Geometry: see drawing. Coordinates: mm, zero at the bounding-box minimum. A direction names the side the tool comes from. Give positions to 0.01 mm unless a question says otherwise; leave off trailing zeros. Write each loop counter-clockwise with the first axis right and the second up, starting at its lowest first coordinate (ties: lowest second). Pieces come first, ordered by that corner, then holes. Notation, with made-up numbers: (20.25, 78.25) -> (52.25, 78.25) arc R20 ccw to (52.25, 106.25) -> close; hole circle Ø10 at (-18.75, 57.5). An arc over 180 degrees is marked (long way). Answer as a JSON object with one key per item and string values. Group by question number.
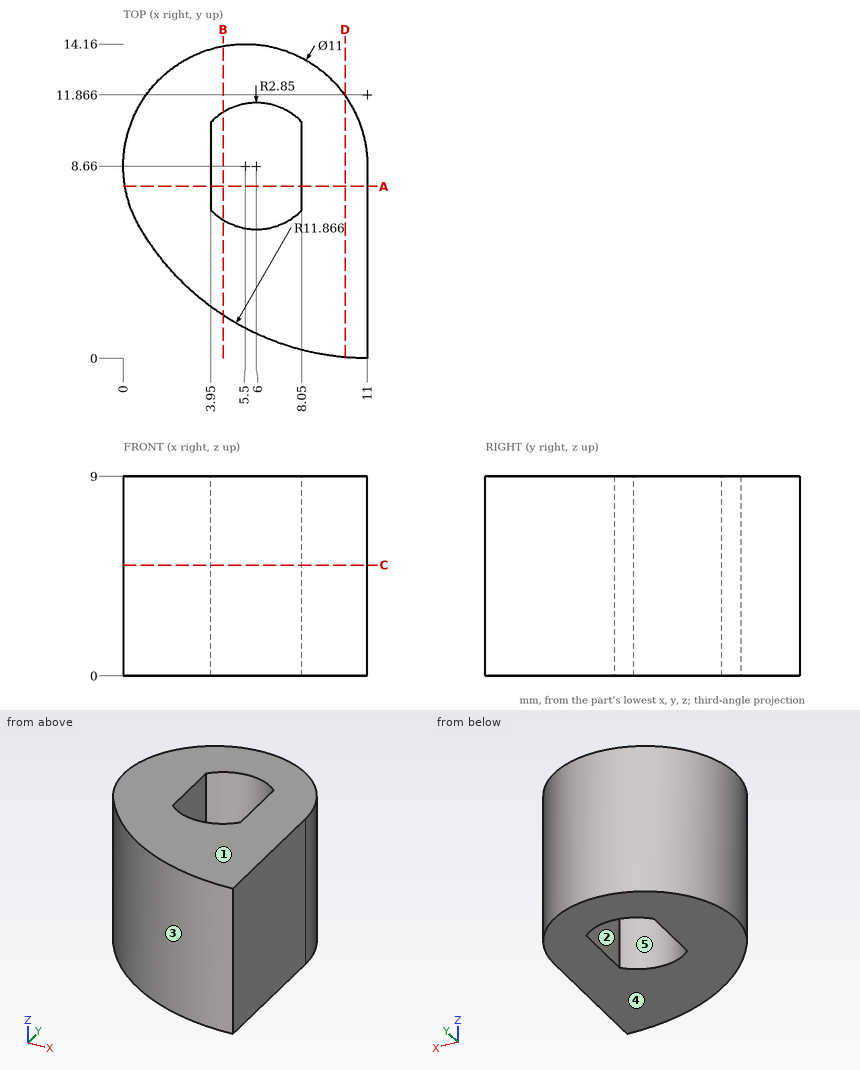
1. Section B-B (x = 4.5). Return the cut outline in (y, z).
2. Section A-A (y = 7.75). Return the cut outline in (x, z).
3. Section D-D (x = 10). Return the cut outline in (y, z), plus the area to 3 significant figures.
4. Reachability of the marked faces 4 and 5 from +Z, -Z, +X, -X, +Y, -Y: full face, straight path, thin tool, end or side. Return the list, or none.
5. Contact query for flat-ended pins moving along their axis: pin 1 Ø3 at (x, z) = (7.5, 2) entering from -Y; pin 2 Ø1.5 at (y, z) = (4, 3.5) entering from -X (1 decimal); pin 3 Ø1 at (x, y) = (2, 2.5) entering from -Z; pin 4 Ø1.5 at (y, z) = (5.5, 4) entering from -X. Output: stop coordinate, or through.
6. Line query: line 1 (Y direction, x = 4.25, z = 1.5); line 2 (Y direction, x = 4.5, z = 6.75); line 3 (X direction, y = 8, z = 5.25). Output: solid intervals per line, ascending.
7. Mould query, pull axis X, two halves, no side actions, for the marked faces 1, 2 and 3. Classes: pulls with the +X half, pulls with the -X half, needs draft (parallel to the pull), parting line crosses it, or undercut.
8. Section C-C (z = 5). Return the cut outline in (x, y).
Working result:
{
 "1": {"outline": "(1.94, 0) -> (6.24, 0) -> (6.24, 9) -> (1.94, 9) -> close; (11.08, 0) -> (14.07, 0) -> (14.07, 9) -> (11.08, 9) -> close"},
 "2": {"outline": "(0.08, 0) -> (3.95, 0) -> (3.95, 9) -> (0.08, 9) -> close; (8.05, 0) -> (11, 0) -> (11, 9) -> (8.05, 9) -> close"},
 "3": {"outline": "(0.04, 0) -> (11.82, 0) -> (11.82, 9) -> (0.04, 9) -> close", "area": "106 mm^2"},
 "4": {"face 4": "-Z, +X, -X, +Y, -Y", "face 5": "+Z, -Z"},
 "5": {"pin 1": "stops at y = 0.17", "pin 2": "stops at x = 1.5", "pin 3": "passes through", "pin 4": "stops at x = 0.56"},
 "6": {"line 1": "y = 2.11 to 6.41, 10.91 to 14.02", "line 2": "y = 1.94 to 6.24, 11.08 to 14.07", "line 3": "x = 0.04 to 3.95, 8.05 to 11"},
 "7": {"face 1": "needs draft", "face 2": "undercut", "face 3": "pulls with the -X half"},
 "8": {"outline": "(0.75, 5.89) arc R11.87 ccw to (11, 0) -> (11, 8.66) arc R5.5 ccw (long way) to start; hole (3.95, 6.68) arc R2.85 ccw to (8.05, 6.68) -> (8.05, 10.64) arc R2.85 ccw to (3.95, 10.64) -> close"}
}
